Here's the drawing with two shaded views (mm, measured from the low corner). I have some questions. A direction names the side the tool comes from. Coordinates: 2 decimals unless noted, no trailing zeros. Write each loop counter-clockwise with the first axis right and the second up, starting at its lowest first coordinate (ties: lowest second). Pieces come first, ordered by that corner, then holes. Notation, with made-up numbers: (16.5, 52) -> (37.5, 52) arc R7 ccw to (37.5, 61) -> close; hole circle Ø10 at (12.25, -17.5). An arc over 180 degrees is marked (long way). Use one line per item in the form item = value.
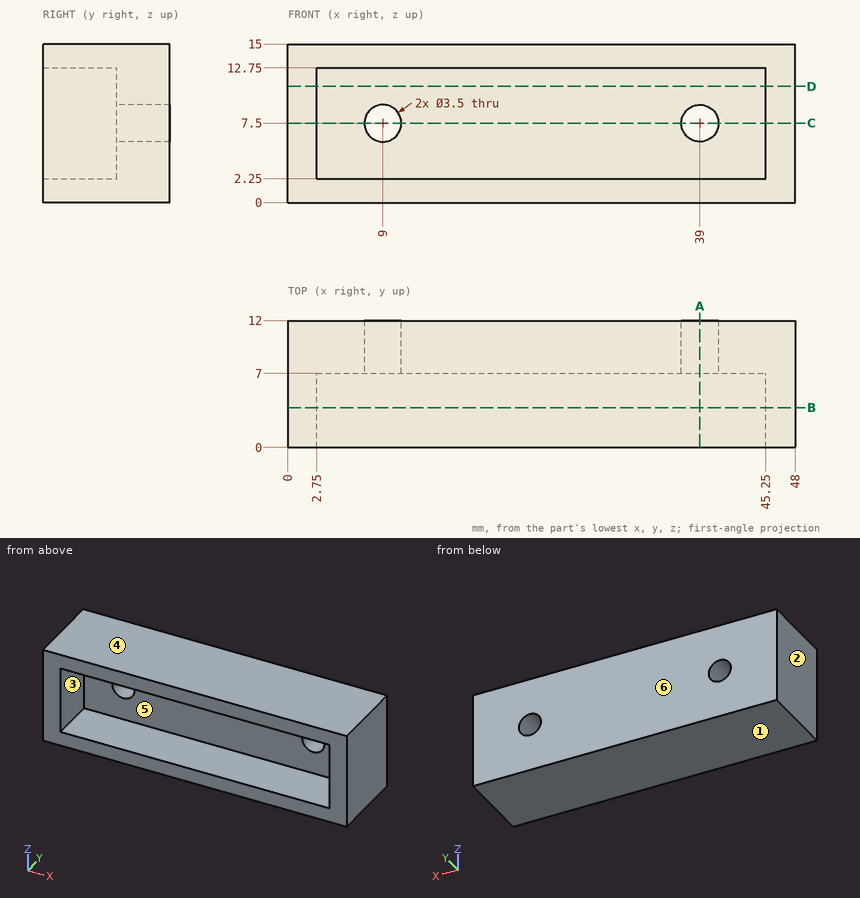
Q1. If I drill on line 1 (Z direction, x = 39, y = 10); line 2 (X direction, y = 4.5, z = 10.75); line 3 (Z direction, x = 16.5, y = 0.75), over which ranges is the centre line in solid material (lowest first)? Write a range as from..to.
Return value:
line_1 = 0..5.75, 9.25..15
line_2 = 0..2.75, 45.25..48
line_3 = 0..2.25, 12.75..15
Q2. Suppose I cut it at A-A (x = 39). Write out the boundary of the cut face in (y, z), then the cut area to 3 significant figures.
Return value:
outline = (0, 0) -> (12, 0) -> (12, 5.75) -> (7, 5.75) -> (7, 2.25) -> (0, 2.25) -> close; (0, 12.75) -> (7, 12.75) -> (7, 9.25) -> (12, 9.25) -> (12, 15) -> (0, 15) -> close
area = 89.0 mm2
Q3. Suppose I cut it at B-B (y = 3.75). Write out the boundary of the cut face in (x, z), then the cut area to 3 significant figures.
Return value:
outline = (0, 0) -> (48, 0) -> (48, 15) -> (0, 15) -> close; hole (2.75, 2.25) -> (45.25, 2.25) -> (45.25, 12.75) -> (2.75, 12.75) -> close
area = 274 mm2
Q4. Thinking about a two-plate mould opening in Z: for the marked faces 1, 2, 3 and 4, which applies, released by +Z, released by -Z, zero draft, split by the parting line, or undercut?
Return value:
face_1 = released by -Z
face_2 = zero draft
face_3 = undercut
face_4 = released by +Z
Q5. For the marked faces 5 and 6, which set-ups out of +Z, -Z, +X, -X, +Y, -Y let a thin tool reach every point of the face, with its end or its side?
Return value:
face_5 = -Y
face_6 = +Z, -Z, +X, -X, +Y
Q6. Will this pin go through, and if not, where does the flat tip stop? pin 1 (5 mm diameter, centred on x = 20, z = 7.5, fed in from -Y).
Return value:
pin_1 = 7
Q7. Suppose I cut it at C-C (z = 7.5). Write out the boundary of the cut face in (x, y).
Return value:
outline = (0, 0) -> (2.75, 0) -> (2.75, 7) -> (7.25, 7) -> (7.25, 12) -> (0, 12) -> close; (10.75, 7) -> (37.25, 7) -> (37.25, 12) -> (10.75, 12) -> close; (40.75, 7) -> (45.25, 7) -> (45.25, 0) -> (48, 0) -> (48, 12) -> (40.75, 12) -> close
Q8. Suppose I cut it at D-D (z = 11). Write out the boundary of the cut face in (x, y).
Return value:
outline = (0, 0) -> (2.75, 0) -> (2.75, 7) -> (45.25, 7) -> (45.25, 0) -> (48, 0) -> (48, 12) -> (0, 12) -> close
